from build123d import *

# Parameters (mm, degrees)
SKETCH1_R           = 1.75
BOSS_EXTRUDE1_DEPTH = 6
CUT_EXTRUDE1_DEPTH  = 2.5


with BuildPart() as part:
    # Sketch1 → Boss-Extrude1 (new body)
    with BuildSketch(Plane(origin=(0, 0, 0), x_dir=(1, 0, 0), z_dir=(0, 1, 0))):
        with BuildLine():
            Line((5, 0), (45, 0))
            ThreePointArc((45, 0), (48.535533906, 1.464466094), (50, 5))
            Line((50, 5), (50, 9))
            ThreePointArc((50, 9), (48.535533906, 12.535533906), (45, 14))
            Line((45, 14), (5, 14))
            ThreePointArc((5, 14), (1.464466094, 12.535533906), (0, 9))
            Line((0, 9), (0, 5))
            ThreePointArc((0, 5), (1.464466094, 1.464466094), (5, 0))
        make_face()
        with Locations((18.25, 7)):
            Circle(SKETCH1_R, mode=Mode.SUBTRACT)
        with Locations((31.75, 7)):
            Circle(SKETCH1_R, mode=Mode.SUBTRACT)
    extrude(amount=BOSS_EXTRUDE1_DEPTH)

    # Sketch2 → Cut-Extrude1 (cut)
    with BuildSketch(Plane(origin=(0, 6, 0), x_dir=(1, 0, 0), z_dir=(0, 1, 0))):
        Polygon((19.83771324, 4.25), (21.425426481, 7), (19.83771324, 9.75), (16.66228676, 9.75), (15.074573519, 7), (16.66228676, 4.25), align=None)
        Polygon((33.33771324, 4.25), (34.925426481, 7), (33.33771324, 9.75), (30.16228676, 9.75), (28.574573519, 7), (30.16228676, 4.25), align=None)
    extrude(amount=-CUT_EXTRUDE1_DEPTH, mode=Mode.SUBTRACT)


solid = part.part
Verification items for the finished model (mm, model axes). A direction names the side the tool comes from. Give positions to 0.01 mm unless a question says otherwise; leave off trailing zeros. Loops run counter-clockwise (first coordinate to the right, second up) from the corner with the lowest first, then second, coordinate; pieces in that order, holes last.
1) Sectioned sample at A-A, the plane y = 4.75. Enter the section's corners in (x, z), then the cut area to 3 significant figures.
2) Depth check by flat-ended pin: pin 1 Ø6 at (x, z) = (13, -7) entering from -Y; pin 2 Ø1.6 at (x, z) = (31.5, -8) entering from +Y. Enter the tip coordinate at first touch or a pass-through.
3) Sectioned sample at C-C, the plane z = -7.75. Enter the section's corners in (x, y), then the cut area to 3 significant figures.
4) Thickness scan on line 1 along X through (y, z) = (2.25, -7); line 2 along X through (y, z) = (2.5, -7.75); line 3 along Z through (x, y) = (18.25, 2.75). Record the ranges inside material, lowest first.
5) Set-up check for faces 1 (the flat face through (20.62, 4.768, -5.606)), 2 (the flat face through (25, 3, 0)): record each of +Z, -Z, +X, -X, +Y, -Y from which the full face is reachable in a straight line by a thin tool's end or side.
6) Sectioned sample at B-B, the plane x = 18.25. Enter the section's corners in (y, z).
7) Sectioned sample at D-D, the plane y = 2.25. Enter the section's corners in (x, z).
8) Draft check along X on faces 3 (the flat face through (25, 6, -7)), 4 (the cylindrical face through (49, 3, -12)), 5 (the flat face through (15.86, 4.77, -5.64)), 6 (the cylindrical face through (1, 3, -2)). Enter one of: pulls with the +X half, pulls with the -X half, needs draft (parallel to the pull), parting line crosses it, or undercut.
Answers:
1. outline: (0, -9) arc R5 ccw to (5, -14) - (45, -14) arc R5 ccw to (50, -9) - (50, -5) arc R5 ccw to (45, 0) - (5, 0) arc R5 ccw to (0, -5) - close; hole (15.07, -7) - (16.66, -9.75) - (19.84, -9.75) - (21.43, -7) - (19.84, -4.25) - (16.66, -4.25) - close; hole (28.57, -7) - (30.16, -9.75) - (33.34, -9.75) - (34.93, -7) - (33.34, -4.25) - (30.16, -4.25) - close
1. area: 626 mm2
2. pin 1: stops at y = 0
2. pin 2: stops at y = 3.5
3. outline: (0, 0) - (16.67, 0) - (16.67, 3.5) - (15.51, 3.5) - (15.51, 6) - (0, 6) - close; (19.83, 0) - (30.17, 0) - (30.17, 3.5) - (29.01, 3.5) - (29.01, 6) - (20.99, 6) - (20.99, 3.5) - (19.83, 3.5) - close; (33.33, 0) - (50, 0) - (50, 6) - (34.49, 6) - (34.49, 3.5) - (33.33, 3.5) - close
3. area: 250 mm2
4. line 1: x = 0 to 16.5, 20 to 30, 33.5 to 50
4. line 2: x = 0 to 16.67, 19.83 to 30.17, 33.33 to 50
4. line 3: z = -14 to -8.75, -5.25 to 0
5. face 1: +Y
5. face 2: +Z, +X, -X, +Y, -Y
6. outline: (0, -14) - (6, -14) - (6, -9.75) - (3.5, -9.75) - (3.5, -8.75) - (0, -8.75) - close; (0, -5.25) - (3.5, -5.25) - (3.5, -4.25) - (6, -4.25) - (6, 0) - (0, 0) - close
7. outline: (0, -9) arc R5 ccw to (5, -14) - (45, -14) arc R5 ccw to (50, -9) - (50, -5) arc R5 ccw to (45, 0) - (5, 0) arc R5 ccw to (0, -5) - close; hole circle Ø3.5 at (18.25, -7); hole circle Ø3.5 at (31.75, -7)
8. face 3: needs draft
8. face 4: pulls with the +X half
8. face 5: undercut
8. face 6: pulls with the -X half
